```python
from build123d import *

# Parameters (mm, degrees)
SKETCH_1_W           = 130
SKETCH_1_H           = 130
EXTRUDE_1_DEPTH      = 5.5
SKETCH_4_R           = 5.4
CUT_EXTRUDE_7_DEPTH  = 4
SKETCH_6_R           = 3.3
CUT_EXTRUDE_8_DEPTH  = 1.5
SKETCH_7_R           = 3.1
CUT_EXTRUDE_9_DEPTH  = 4.2
SKETCH_8_R           = 1.6
CUT_EXTRUDE_10_DEPTH = 2.3


with BuildPart() as part:
    # 草图1 → 凸台-拉伸1 (new body)
    with BuildSketch(Plane(origin=(0, 0, 0), x_dir=(1, 0, 0), z_dir=(0, 1, 0))):
        with Locations((65, 65)):
            Rectangle(SKETCH_1_W, SKETCH_1_H)
    extrude(amount=EXTRUDE_1_DEPTH)

    # 草图4 → 切除-拉伸7 (cut)
    with BuildSketch(Plane(origin=(0, 5.5, 0), x_dir=(1, 0, 0), z_dir=(0, 1, 0))):
        with Locations((10, 120)):
            Circle(SKETCH_4_R)
        with Locations((120, 120)):
            Circle(SKETCH_4_R)
        with Locations((10, 10)):
            Circle(SKETCH_4_R)
        with Locations((120, 10)):
            Circle(SKETCH_4_R)
    extrude(amount=-CUT_EXTRUDE_7_DEPTH, mode=Mode.SUBTRACT)

    # 草图6 → 切除-拉伸8 (cut)
    with BuildSketch(Plane(origin=(0, 1.5, 0), x_dir=(1, 0, 0), z_dir=(0, 1, 0))):
        with Locations((10, 120)):
            Circle(SKETCH_6_R)
        with Locations((119.916006429, 119.916006429)):
            Circle(SKETCH_6_R)
        with Locations((10, 10)):
            Circle(SKETCH_6_R)
        with Locations((120, 9.916006429)):
            Circle(SKETCH_6_R)
    extrude(amount=-CUT_EXTRUDE_8_DEPTH, mode=Mode.SUBTRACT)

    # 草图7 → 切除-拉伸9 (cut)
    with BuildSketch(Plane.XZ):
        with Locations((20, -40)):
            Circle(SKETCH_7_R)
        with Locations((20, -75)):
            Circle(SKETCH_7_R)
        with Locations((109.5, -38.5)):
            Circle(SKETCH_7_R)
        with Locations((109.5, -88.5)):
            Circle(SKETCH_7_R)
    extrude(amount=-CUT_EXTRUDE_9_DEPTH, mode=Mode.SUBTRACT)

    # 草图8 → 切除-拉伸10 (cut, through all)
    with BuildSketch(Plane.XZ.offset(-4.2)):
        with Locations((20, -40)):
            Circle(SKETCH_8_R)
        with Locations((20, -75)):
            Circle(SKETCH_8_R)
        with Locations((109.5, -38.5)):
            Circle(SKETCH_8_R)
        with Locations((109.5, -88.5)):
            Circle(SKETCH_8_R)
    extrude(amount=-CUT_EXTRUDE_10_DEPTH, mode=Mode.SUBTRACT)


solid = part.part
```
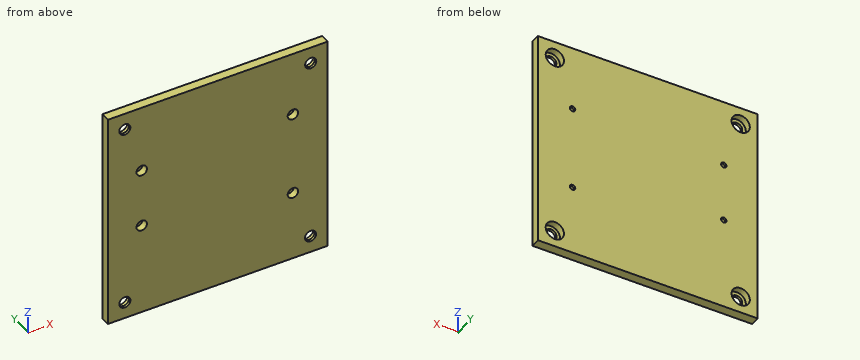
Source: CAD feature listing. Evaluate the final solid. Frame: model axes, mm. Round coordinates to 2 decimals unless told otherwise and drop trailing zeros. Loops run counter-clockwise (first coordinate to the right, second up) from the corner with the lowest first, then second, coordinate; pieces in that order, holes last. Notation, with made-up numbers: M -18,50.25 L 24,50.25 A19 cw 24,72.25 Z; hole C 83.5,23.5 d1. An arc over 180 degrees is marked long. Use a Markdown table: item, result. Add a question column.
1. Contact query for flat-ended pins moving along their axis: pin 1 (8.5 mm diameter, centred on x = 10, z = -10, fed in from +Y); pin 2 (12.5 mm diameter, centred on x = 10, z = -120, fed in from -Y); pin 3 (3 mm diameter, centred on x = 20, z = -74.5, fed in from -Y). Output: stop coordinate, or through.
2. Ray query, line 1 along Z through (x, y) = (10, 0.7); line 2 along Z through (x, y) = (20, 1.4); line 3 along X through (y, z) = (2.9, -120). Return the intervals inside material, ascending. Write a range as [from, to].
3. Cut plane A-A, the plane x = 10. Output: boundary loops of the cut face in (y, z).
4. Cut plane B-B, the plane x = 109.5. Output: boundary loops of the cut face in (y, z).
Solution:
| question | item | result |
|---|---|---|
| 1 | pin 1 | stops at y = 1.5 |
| 1 | pin 2 | stops at y = 0 |
| 1 | pin 3 | stops at y = 4.2 |
| 2 | line 1 | z = [-130, -123.3], [-116.7, -13.3], [-6.7, 0] |
| 2 | line 2 | z = [-130, -78.1], [-71.9, -43.1], [-36.9, 0] |
| 2 | line 3 | x = [0, 4.6], [15.4, 114.6], [125.4, 130] |
| 3 | outline | M 0,-130 L 5.5,-130 L 5.5,-125.4 L 1.5,-125.4 L 1.5,-123.3 L 0,-123.3 Z; M 0,-116.7 L 1.5,-116.7 L 1.5,-114.6 L 5.5,-114.6 L 5.5,-15.4 L 1.5,-15.4 L 1.5,-13.3 L 0,-13.3 Z; M 0,-6.7 L 1.5,-6.7 L 1.5,-4.6 L 5.5,-4.6 L 5.5,0 L 0,0 Z |
| 4 | outline | M 0,-130 L 5.5,-130 L 5.5,-90.1 L 4.2,-90.1 L 4.2,-91.6 L 0,-91.6 Z; M 0,-85.4 L 4.2,-85.4 L 4.2,-86.9 L 5.5,-86.9 L 5.5,-40.1 L 4.2,-40.1 L 4.2,-41.6 L 0,-41.6 Z; M 0,-35.4 L 4.2,-35.4 L 4.2,-36.9 L 5.5,-36.9 L 5.5,0 L 0,0 Z |
